```python
from build123d import *

# Parameters (mm, degrees)
SKETCH1_W           = 584.2
SKETCH1_H           = 584.2
SKETCH1_R           = 3.175
BOSS_EXTRUDE1_DEPTH = 6.35
FILLET1_R           = 12.7


with BuildPart() as part:
    # Sketch1 → Boss-Extrude1 (new body)
    with BuildSketch(Plane.XY):
        Rectangle(SKETCH1_W, SKETCH1_H)
        with Locations((-266.7, 139.7)):
            Circle(SKETCH1_R, mode=Mode.SUBTRACT)
        with Locations((-88.9, 139.7)):
            Circle(SKETCH1_R, mode=Mode.SUBTRACT)
        with Locations((88.9, 139.7)):
            Circle(SKETCH1_R, mode=Mode.SUBTRACT)
        with Locations((266.7, 139.7)):
            Circle(SKETCH1_R, mode=Mode.SUBTRACT)
        with Locations((-88.9, 158.75)):
            Circle(SKETCH1_R, mode=Mode.SUBTRACT)
        with Locations((88.9, 158.75)):
            Circle(SKETCH1_R, mode=Mode.SUBTRACT)
        with Locations((266.7, 158.75)):
            Circle(SKETCH1_R, mode=Mode.SUBTRACT)
        with Locations((-266.7, 158.75)):
            Circle(SKETCH1_R, mode=Mode.SUBTRACT)
        with BuildLine():
            Line((-228.6, 273.05), (-76.2, 273.05))
            ThreePointArc((-76.2, 273.05), (-57.15, 254), (-76.2, 234.95))
            Line((-76.2, 234.95), (-228.6, 234.95))
            ThreePointArc((-228.6, 234.95), (-247.65, 254), (-228.6, 273.05))
        make_face(mode=Mode.SUBTRACT)
        with BuildLine():
            Line((76.2, 273.05), (228.6, 273.05))
            ThreePointArc((228.6, 273.05), (247.65, 254), (228.6, 234.95))
            Line((228.6, 234.95), (76.2, 234.95))
            ThreePointArc((76.2, 234.95), (57.15, 254), (76.2, 273.05))
        make_face(mode=Mode.SUBTRACT)
    extrude(amount=BOSS_EXTRUDE1_DEPTH)

    # Fillet1
    fillet1_edges = [part.edges().sort_by_distance(p)[0] for p in [
        (292.1, -292.1, 3.175),
        (-292.1, -292.1, 3.175),
        (-292.1, 292.1, 3.175),
        (292.1, 292.1, 3.175),
    ]]
    fillet(fillet1_edges, radius=FILLET1_R)


solid = part.part
```
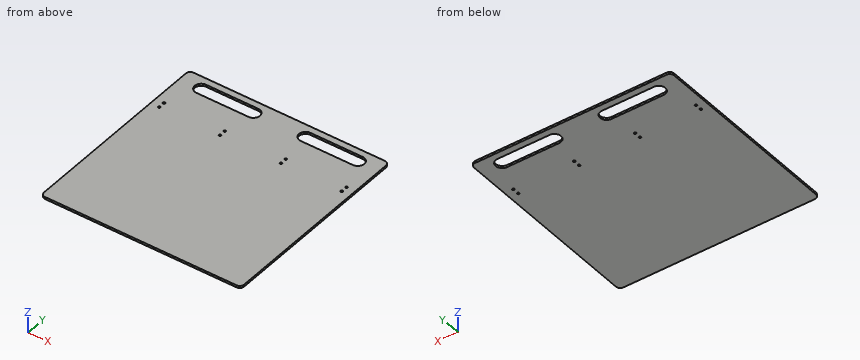
Verification items for the finished model (mm, model axes). Coordinates: 2 decimals unless noted, no trailing zeros. Write each loop counter-clockwise with the first axis right and the second up, starting at its lowest first coordinate (ties: lowest second). Pieces come first, ordered by that corner, then holes. Notation, with made-up numbers: (83, 33) - (104, 33) arc R23 cw to (104, 54) - close; hole circle Ø4 at (-35, 32). An arc over 180 degrees is marked (long way). Write item = value, one per line.
Q1. Cross-section at C-C (y = 254). Enter the section's corners in (x, z).
Answer:
outline = (-292.1, 0) - (-247.65, 0) - (-247.65, 6.35) - (-292.1, 6.35) - close; (-57.15, 0) - (57.15, 0) - (57.15, 6.35) - (-57.15, 6.35) - close; (247.65, 0) - (292.1, 0) - (292.1, 6.35) - (247.65, 6.35) - close
Q2. Go/stop test with flat-tipped pins: pin 1 Ø5 at (x, y) = (266.7, 158.75) entering from +Z; pin 2 Ø8 at (x, y) = (-10.5, 47) entering from -Z. Record where each tip stops, or that it passes through.
Answer:
pin_1 = through
pin_2 = 0
Q3. Material ranges on L1, parallel to X at y = 139.7, z = 1.75 (3 decimals); L2, parallel to Y at x = -266.7, z = 1.5 (3 decimals); L3, parallel to Y at x = -88, z = 3.75, recorded low to high. Write a range as from..to.
Answer:
L1 = -292.1..-269.875, -263.525..-92.075, -85.725..85.725, 92.075..263.525, 269.875..292.1
L2 = -292.1..136.525, 142.875..155.575, 161.925..292.1
L3 = -292.1..136.66, 142.74..155.71, 161.79..234.95, 273.05..292.1
Q4. Cross-section at A-A (x = 169.5). Enter the section's corners in (y, z).
Answer:
outline = (-292.1, 0) - (234.95, 0) - (234.95, 6.35) - (-292.1, 6.35) - close; (273.05, 0) - (292.1, 0) - (292.1, 6.35) - (273.05, 6.35) - close
Q5. Cross-section at B-B (z = 2.75). Give the number of separate pieces and of enclosed holes in the cut face, plus the area to 3 significant figures.
Answer:
separate_pieces = 1
enclosed_holes = 10
area = 327,000 mm²
